CAD build for the part. Positions are in the model's coordinates, mm. A direction names the side the tool comes from. Give positions to 0.01 mm unless a question says otherwise; leave off trailing zeros. Loops run counter-clockwise (first coordinate to the right, second up) from the corner with the lowest first, then second, coordinate; pieces in that order, holes last. Notation, with made-up numbers: M 85.5,6 L 139.5,6 A21 cw 139.5,19 Z; hole C -4,72.25 d9. An arc over 180 degrees is marked long. One line per question, with ' | ' between items.
```python
from build123d import *

# Parameters (mm, degrees)
PAD_DEPTH        = 10
SKETCH001_R      = 3.05
POCKET_DEPTH     = 10.001
FILLET_R         = 2
FILLET001_R      = 2
HOLE_D           = 6.6
HOLE_DEPTH       = 25
HOLE_CBORE_D     = 11
HOLE_CBORE_DEPTH = 6.4


with BuildPart() as part:
    # Sketch → Pad (new body)
    with BuildSketch(Plane.XY):
        with BuildLine():
            Line((-45.5, 24), (45.5, 24))
            ThreePointArc((48.5, 21), (47.62132, 23.12132), (45.5, 24))
            Line((48.5, 21), (48.5, -21))
            ThreePointArc((45.5, -24), (47.62132, -23.12132), (48.5, -21))
            Line((45.5, -24), (-45.5, -24))
            ThreePointArc((-48.5, -21), (-47.62132, -23.12132), (-45.5, -24))
            Line((-48.5, -21), (-48.5, 21))
            ThreePointArc((-45.5, 24), (-47.62132, 23.12132), (-48.5, 21))
        make_face()
        with BuildLine():
            ThreePointArc((40.55, 13), (37.5, 16.05), (34.45, 13))
            Line((34.45, 13), (34.45, -13))
            ThreePointArc((34.45, -13), (37.5, -16.05), (40.55, -13))
            Line((40.55, -13), (40.55, 13))
        make_face(mode=Mode.SUBTRACT)
        with BuildLine():
            ThreePointArc((-34.45, 13), (-37.5, 16.05), (-40.55, 13))
            Line((-40.55, 13), (-40.55, -13))
            ThreePointArc((-40.55, -13), (-37.5, -16.05), (-34.45, -13))
            Line((-34.45, -13), (-34.45, 13))
        make_face(mode=Mode.SUBTRACT)
    extrude(amount=PAD_DEPTH)

    # Sketch001 (on Face18 of Pad) → Pocket (cut, through all)
    with BuildSketch(Plane.XY.offset(10)):
        with Locations((-12.5, 12.5)):
            Circle(SKETCH001_R)
        with Locations((12.5, 12.5)):
            Circle(SKETCH001_R)
        with Locations((-12.5, -12.5)):
            Circle(SKETCH001_R)
        with Locations((12.5, -12.5)):
            Circle(SKETCH001_R)
    extrude(amount=-POCKET_DEPTH, mode=Mode.SUBTRACT)

    # Fillet
    fillet_edges = [part.edges().sort_by_distance(p)[0] for p in [
        (0, -24, 10),
    ]]
    fillet(fillet_edges, radius=FILLET_R)

    # Fillet001
    fillet001_edges = [part.edges().sort_by_distance(p)[0] for p in [
        (0, -24, 0),
    ]]
    fillet(fillet001_edges, radius=FILLET001_R)

    # Hole
    with Locations(Plane.XY.offset(10)):
        with Locations((12.5, 0), (-12.5, 0)):
            CounterBoreHole(HOLE_D / 2, HOLE_CBORE_D / 2, HOLE_CBORE_DEPTH, depth=HOLE_DEPTH)


solid = part.part
```
Item 1: Drop flat-ended pins along their axis: P1, Ø5.5, axis at x = -12.5, y = -12.5, coming from the +Z side; P2, Ø3.5, axis at x = -12.5, y = -2, coming from the +Z side. Give the stop position or say it passes through.
Conclusion:
P1: through | P2: z = 3.6
Item 2: Drill centre lines: line 1 along Y through (x, z) = (-12.5, 1.85); line 2 along Y through (x, z) = (12.5, 5); line 3 along X through (y, z) = (2.5, 6.5). Where is each one in solid material? Low to high. Write a range as [from, to].
Conclusion:
line 1: [-23.99, -15.55], [-9.45, -3.3], [3.3, 9.45], [15.55, 23.99] | line 2: [-24, -15.55], [-9.45, -5.5], [5.5, 9.45], [15.55, 24] | line 3: [-48.5, -40.55], [-34.45, -17.4], [-7.6, 7.6], [17.4, 34.45], [40.55, 48.5]
Item 3: 3-axis set-ups, long thin cutter, end or side, ignore diameter. For faces 4 (the cylindrical face through (37.43, -16.05, 4.93)), 5 (the flat face through (48.5, 0, 5)), 6 (the flat face through (-9, 0, 3.6)): which of +Z, -Z, +X, -X, +Y, -Y reach the whole face in a straight line?
Conclusion:
face 4: +Z, -Z | face 5: +Z, -Z, +X, +Y, -Y | face 6: +Z
Item 4: Mould opens along Y. For faces 1 (the cylindrical face through (47.6, -23.14, 4.96)), 2 (the cylindrical face through (47.9, -0.29, 0.57)), 3 (the cylindrical face through (10.25, 14.56, 5.07)) say: pulls with the +Y half, pulls with the -Y half, needs draft (parallel to the pull), parting line crosses it, or undercut.
Conclusion:
face 1: pulls with the -Y half | face 2: needs draft | face 3: undercut
Item 5: Saw through at C-C on y = -6.5. Give the cut face in (x, z).
Conclusion:
outline: M -48.5,2 A2 ccw -46.5,0 L -40.55,0 L -40.55,10 L -46.5,10 A2 ccw -48.5,8 Z; M -34.45,0 L 34.45,0 L 34.45,10 L -34.45,10 Z; M 40.55,0 L 46.5,0 A2 ccw 48.5,2 L 48.5,8 A2 ccw 46.5,10 L 40.55,10 Z
Item 6: Saw through at B-B on y = 0. State how many separate pieces and enclosed holes the cut face has, and give its area (3 significant figures).
Conclusion:
separate pieces: 5 | enclosed holes: 0 | area: 656 mm²
Item 7: Saw through at A-A on x = 37.5. Give the cut face in (y, z).
Conclusion:
outline: M -24,2 A2 ccw -22,0 L -16.05,0 L -16.05,10 L -22,10 A2 ccw -24,8 Z; M 16.05,0 L 22,0 A2 ccw 24,2 L 24,8 A2 ccw 22,10 L 16.05,10 Z
